Print and shaded views of the part. All mm, measured from the part's lowest x, y and z. Coordinates: 2 decimals unless noted, no trailing zeros. Write item = value, one per line. Start each with the question number.
Q1. Wall check: line 1 (Z direction, x = 19, y = 285) (1 decimal); line 2 (X direction, y = 374, z = 19.5); line 3 (Z direction, x = 21, y = 315) (1 decimal). Give the ranges that are in metal, low to high. Write a range as from..to.
Q2. Flat gauge pin, fed straight in: pin 1 (2 mm diameter, centred on y = 314.5, z = 52.5, fed in from -X). Where does the tip first touch, or does it go through?
Q3. Cut at A-A, the plane y = 211. Give the number of separate pieces and of enclosed holes in the cut face, plus the area to 3 significant figures.
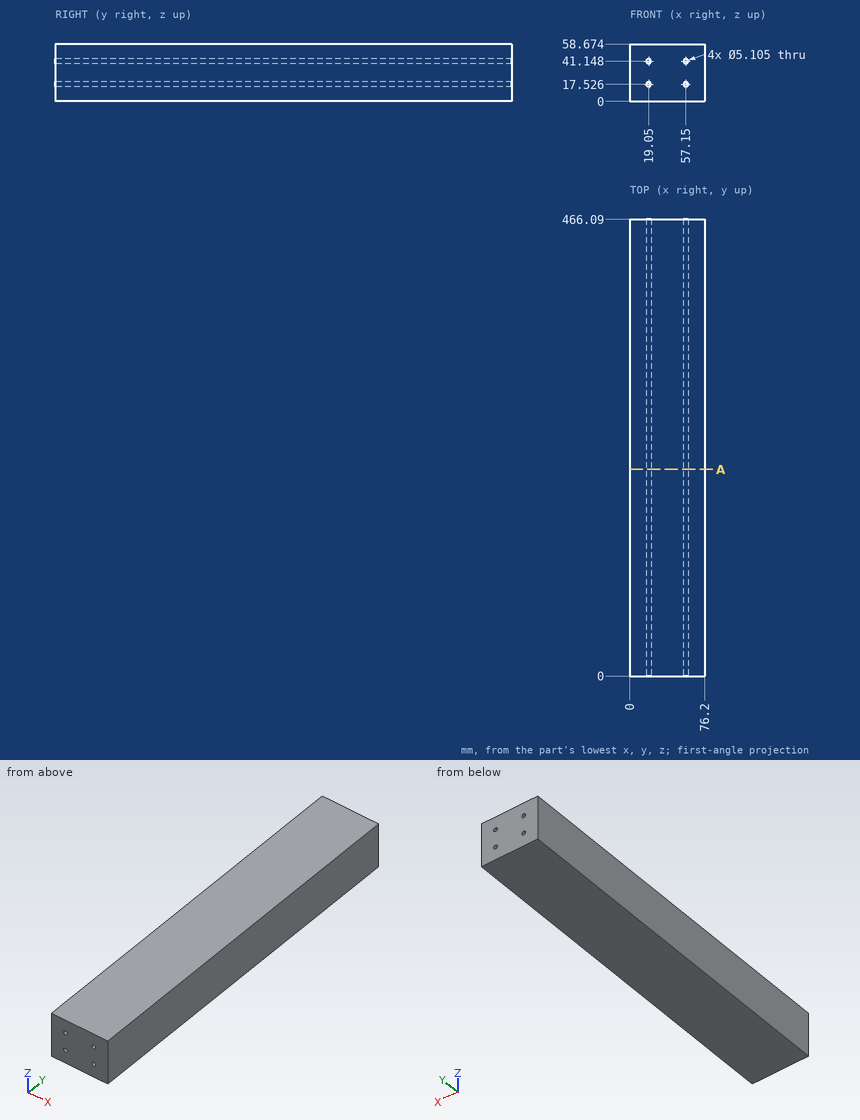
Here are the results:
q1.line_1 = 0..15, 20.1..38.6, 43.7..58.7
q1.line_2 = 0..17.43, 20.67..55.53, 58.77..76.2
q1.line_3 = 0..15.9, 19.2..39.5, 42.8..58.7
q2.pin_1 = 0
q3.separate_pieces = 1
q3.enclosed_holes = 4
q3.area = 4,390 mm²
